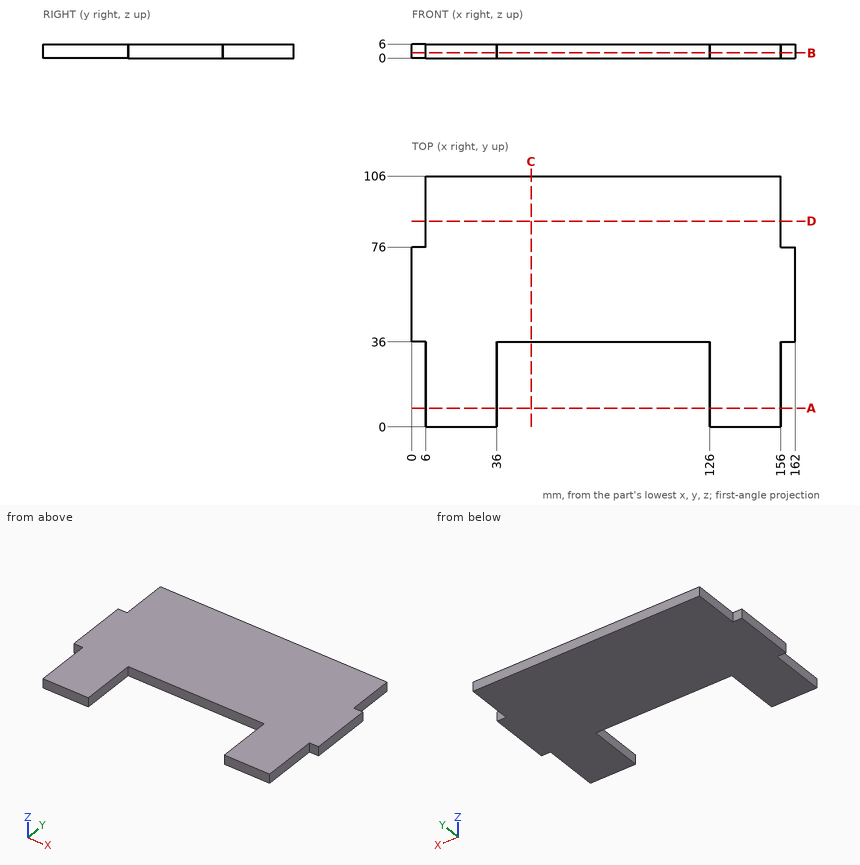
Could you check a few things on this drawing? It's one solid part, dimensions in mm from its lowest x, y, z. Give positions to 0.01 mm unless a question says otherwise; leave off trailing zeros. Loops run counter-clockwise (first coordinate to the right, second up) from the corner with the lowest first, then second, coordinate; pieces in that order, holes last. Notation, with made-up numbers: (68.5, -9) -> (98.5, -9) arc R10 cw to (98.5, -2) -> close; hole circle Ø5 at (-26.75, 16). An arc over 180 degrees is marked (long way). Answer as CSV lines item,"result". Start each with the question number.
(1) If we section it at C-C on x = 50.5: Write out the boundary of the cut face in (y, z).
(2) If we section it at A-A on y = 8: Write out the boundary of the cut face in (x, z).
(3) If we section it at B-B on z = 2.2: Write out the boundary of the cut face in (x, y), then the cut area to 3 significant figures.
(4) I need wall thicknesses on probe 1 along X at (y, z) = (21, 1.55); probe 2 along Y at (x, z) = (71, 4.25); probe 3 along X at (y, z) = (101.5, 5.15). Which ranges of each line are inside material? Lowest first, please.
(5) If we section it at D-D on y = 87: Write out the boundary of the cut face in (x, z).
(6) I'm going to push flat-ended pins straight in: pin 1 Ø1.8 at (y, z) = (96.5, 4.5) entering from +X; pin 2 Ø1.8 at (y, z) = (12.5, 4.5) entering from -X; pin 3 Ø3 at (x, z) = (80, 2.5) entering from -Y. Where does each tip first touch, or does it pass through?
Computed:
1,outline,"(36, 0) -> (106, 0) -> (106, 6) -> (36, 6) -> close"
2,outline,"(6, 0) -> (36, 0) -> (36, 6) -> (6, 6) -> close; (126, 0) -> (156, 0) -> (156, 6) -> (126, 6) -> close"
3,outline,"(0, 36) -> (6, 36) -> (6, 0) -> (36, 0) -> (36, 36) -> (126, 36) -> (126, 0) -> (156, 0) -> (156, 36) -> (162, 36) -> (162, 76) -> (156, 76) -> (156, 106) -> (6, 106) -> (6, 76) -> (0, 76) -> close"
3,area,"13,100 mm2"
4,probe 1,"x = 6 to 36, 126 to 156"
4,probe 2,"y = 36 to 106"
4,probe 3,"x = 6 to 156"
5,outline,"(6, 0) -> (156, 0) -> (156, 6) -> (6, 6) -> close"
6,pin 1,"stops at x = 156"
6,pin 2,"stops at x = 6"
6,pin 3,"stops at y = 36"
